```python
from build123d import *

# Parameters (mm, degrees)
CROQUIS1_R              = 9.5
SALIENTE_EXTRUIR1_DEPTH = 6
CROQUIS2_R              = 1.5
CORTAR_EXTRUIR1_DEPTH   = 6
REDONDEO1_R             = 1


with BuildPart() as part:
    # Croquis1 → Saliente-Extruir1 (new body)
    with BuildSketch(Plane(origin=(0, 0, 0), x_dir=(1, 0, 0), z_dir=(0, 1, 0))):
        with BuildLine():
            Line((-25.374701647, 20.783734094), (-29.767291136, 10.621141392))
            ThreePointArc((-29.767291136, 10.621141392), (-29.942112128, 10.153967486), (-30.069514751, 9.671699501))
            ThreePointArc((-30.069514751, 9.671699501), (-30.150557328, 9.157351254), (-30.17766953, 8.637363805))
            Line((-30.17766953, 8.637363805), (-30.17766953, -16))
            Line((-30.17766953, -16), (-42, -16))
            Line((-42, -16), (-42, -21))
            Line((-42, -21), (-29.5, -21))
            Line((-29.5, -21), (-29.5, -36))
            Line((-29.5, -36), (-18.5, -36))
            Line((-18.5, -36), (-18.5, -21))
            Line((-18.5, -21), (-6, -21))
            Line((-6, -21), (-6, -16))
            Line((-6, -16), (-17.67766953, -16))
            Line((-17.67766953, -16), (-17.67766953, 4.671699501))
            ThreePointArc((-17.67766953, 4.671699501), (-16.213203436, 8.207233407), (-12.67766953, 9.671699501))
            Line((-12.67766953, 9.671699501), (-8.928571429, 9.671699501))
            ThreePointArc((-8.928571429, 9.671699501), (-4.713647249, 31.429321655), (-24.974516609, 22.448404084))
            ThreePointArc((-24.974516609, 22.448404084), (-25.102827296, 21.598812807), (-25.374701647, 20.783734094))
        make_face()
        with Locations(Location((-12.5, 21.650635095, 0), (0, 0, 270))):
            Circle(CROQUIS1_R, mode=Mode.SUBTRACT)
    extrude(amount=SALIENTE_EXTRUIR1_DEPTH)

    # Croquis2 → Cortar-Extruir1 (cut)
    with BuildSketch(Plane.XY.offset(21)):
        with Locations((-36, 3)):
            Circle(CROQUIS2_R)
        with Locations((-12, 3)):
            Circle(CROQUIS2_R)
    extrude(amount=-CORTAR_EXTRUIR1_DEPTH, mode=Mode.SUBTRACT)

    # Redondeo1
    redondeo1_edges = [part.edges().sort_by_distance(p)[0] for p in [
        (-24, 0, 36),
        (-18.5, 3, 36),
        (-29.5, 3, 36),
        (-24, 6, 36),
    ]]
    fillet(redondeo1_edges, radius=REDONDEO1_R)


solid = part.part
```
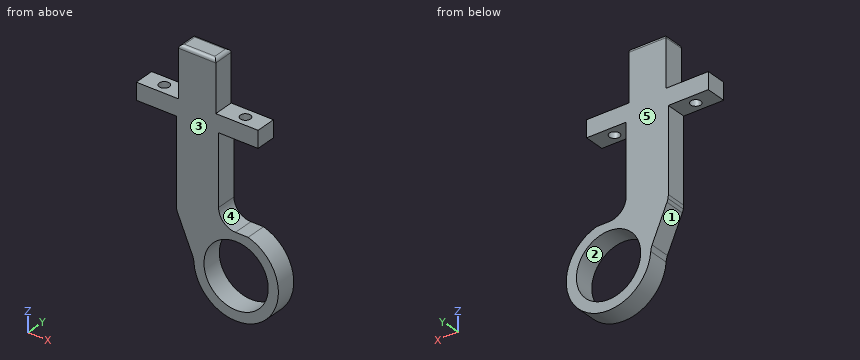
Verification items for the finished model (mm, model axes). Face numbers are marked on the shaded views. A direction names the side the tool comes from. Give positions to 0.01 mm unless a question says otherwise; leave off trailing zeros. Write each loop counter-clockwise with the first axis right and the second up, starting at its lowest first coordinate (ties: lowest second). Pieces come first, ordered by that corner, then holes. Notation, with made-up numbers: M -7,84 L -1,84 A13 cw -1,107 Z; hole C 38,-10 d7. An arc over 180 degrees is marked long. One line per question, with ' | ' between items.
1) Section check D-D on z = 14. Enter the section's corners in (x, y), plus the area to 3 significant figures.
Result:
outline: M -30.18,0 L -17.68,0 L -17.68,6 L -30.18,6 Z | area: 75.0 mm2
2) Mould release check, pull along X, two halves, no side actions. Record for the marked faces 1, 2 and 3: released by +X, released by -X, zero draft, split by the parting line, or undercut.
Result:
face 1: released by -X | face 2: undercut | face 3: zero draft
3) Gauge pin test, flat ends, axial feed: pin 1 Ø2.5 at (x, y) = (-12, 3) entering from +Z; pin 2 Ø1.5 at (y, z) = (3.5, -7.5) entering from -X; pin 3 Ø1.8 at (y, z) = (3.5, 30) entering from -X. Record the tip position at first contact, or that the pin passes through.
Result:
pin 1: stops at z = -9.64 | pin 2: stops at x = -30.18 | pin 3: stops at x = -29.5
4) Section check A-A on y = 3. Enter the section's corners in (x, z), plus the area to 3 significant figures.
Result:
outline: M -42,16 L -37.5,16 L -37.5,21 L -42,21 Z; M -34.5,16 L -30.18,16 L -30.18,-8.64 A5 ccw -29.77,-10.62 L -25.37,-20.78 A5 cw -24.97,-22.45 A12.5 ccw long -8.93,-9.67 L -12.68,-9.67 A5 cw -17.68,-4.67 L -17.68,16 L -13.5,16 L -13.5,21 L -18.5,21 L -18.5,35 A1 ccw -19.5,36 L -28.5,36 A1 ccw -29.5,35 L -29.5,21 L -34.5,21 Z; M -10.5,16 L -6,16 L -6,21 L -10.5,21 Z; hole C -12.5,-21.65 d19 | area: 905 mm2
5) Set-up check for the marked faces 4 and 5: record each of +Z, -Z, +X, -X, +Y, -Y from which the full face is reachable in a straight line by a thin tool's end or side.
Result:
face 4: +X, +Y, -Y | face 5: +Z, -Z, +X, -X, +Y
6) Thickness scan on line 1 along Z through (x, y) = (-15, 1.5); line 2 along Z through (x, y) = (-9, 4.3); line 3 along Z through (x, y) = (-33, 0.8). Record the ranges inside material, lowest first. Write a range as [from, to].
Result:
line 1: z = [-33.9, -30.82], [-12.49, -9.1], [16, 21] | line 2: z = [-33.65, -30.48], [-12.82, -9.67], [16, 21] | line 3: z = [16, 21]
7) Section check C-C on x = -7.5. Enter the section's corners in (y, z), plus the area to 3 significant figures.
Result:
outline: M 0,-33.11 L 6,-33.11 L 6,-29.73 L 0,-29.73 Z; M 0,-13.57 L 6,-13.57 L 6,-10.19 L 0,-10.19 Z; M 0,16 L 6,16 L 6,21 L 0,21 Z | area: 70.5 mm2
8) Section check B-B on x = -36. Enter the section's corners in (y, z).
Result:
outline: M 0,16 L 1.5,16 L 1.5,21 L 0,21 Z; M 4.5,16 L 6,16 L 6,21 L 4.5,21 Z
